Check sheet for the modelled part. Datum: model origin and axes. Units: mm. Round coordinates to 2 decimals unless told otherwise and drop trailing zeros. Order: outer loops, then holes, each group sorted by start corner. A loop starts at its lowest first (then second) coordinate and runs counter-clockwise, first axis right, second up. Notation, with made-up numbers: M 65,38.5 L 85,38.5 A18 cw 85,47.5 Z; hole C -39.75,-37 d5. An arc over 180 degrees is marked long. One line per item, written item: value. Start each with the question number.
(1) Release check for a two-part mould opening along X. For faces 1 (the face through (-3.563, 1.772, -0.791)), 2 (the face through (-2.4, 0, 0.8)), 3 (the face through (0.71, 2.29, 2.24)), 4 (the face through (8.406, 3.575, 3.006)) record: released by +X, released by -X, zero draft, split by the parting line, or undercut.
(2) Thickness scan on L1, parallel to X at y = 3.25, z = 0; L2, parallel to X at y = 2.2, z = 0; L3, parallel to Y at x = 4, z = 2. Record the ranges inside material, lowest first.
(3) Cross-section at D-D, the plane z = 2. Enter the section's corners in (x, y).
(4) Cross-section at C-C, the plane y = 3. Enter the section's corners in (x, z), and give its area (3 significant figures).
(5) Depth check by flat-ended pin: pin 1 Ø3.5 at (x, z) = (8, -1) entering from -Y; pin 2 Ø1 at (y, z) = (1.5, 0.5) entering from -X; pin 3 Ø2 at (x, y) = (4, 1.5) entering from +Z; pin 4 Ø2 at (y, z) = (4, 1.5) entering from +X. Enter the tip coordinate at first touch or a pass-through.
(6) Cross-section at A-A, the plane x = 0. Enter the section's corners in (y, z).
(7) Cross-section at B-B, the plane z = 0. Enter the section's corners in (x, y).
from build123d import *

# Parameters (mm, degrees)
SKETCH1_R           = 3.65
SKETCH1_R_2         = 2.35
BOSS_EXTRUDE1_DEPTH = 4.64
BOSS_EXTRUDE2_START = -2.1
BOSS_EXTRUDE2_DEPTH = 2.1


with BuildPart() as part:
    # Sketch1 → Boss-Extrude1 (new body)
    with BuildSketch(Plane(origin=(0, 0, 0), x_dir=(1, 0, 0), z_dir=(0, 1, 0))):
        with Locations(Location((0, 0, 0), (0, 0, 270))):
            Circle(SKETCH1_R)
        with Locations(Location((0, 0, 0), (0, 0, 270))):
            Circle(SKETCH1_R_2, mode=Mode.SUBTRACT)
    extrude(amount=BOSS_EXTRUDE1_DEPTH)

    # Sketch2 → Boss-Extrude2 (add)
    with BuildSketch(Plane(origin=(0, 4.64, 0), x_dir=(1, 0, 0), z_dir=(0, 1, 0)).offset(BOSS_EXTRUDE2_START)):
        with BuildLine():
            Line((0.283385093, 3.638982397), (16.303738301, 2.391400302))
            ThreePointArc((16.303738301, 2.391400302), (18.500063478, 0), (16.303738301, -2.391400302))
            Line((16.303738301, -2.391400302), (0.283385093, -3.638982397))
            ThreePointArc((0.283385093, -3.638982397), (3.65, 0), (0.283385093, 3.638982397))
        make_face()
    extrude(amount=BOSS_EXTRUDE2_DEPTH)


solid = part.part
Values found:
1. face 1: split by the parting line
1. face 2: zero draft
1. face 3: undercut
1. face 4: released by +X
2. L1: -3.65 to -2.35, 2.35 to 18.5
2. L2: -3.65 to -2.35, 2.35 to 3.65
2. L3: 2.54 to 4.64
3. outline: M -3.05,0 L -1.23,0 L -1.23,4.64 L -3.05,4.64 Z; M 1.23,0 L 3.05,0 L 3.05,2.54 L 17.43,2.54 L 17.43,4.64 L 1.23,4.64 Z
4. outline: M 0.28,-3.64 L 16.3,-2.39 A2.4 ccw 16.3,2.39 L 0.28,3.64 A3.65 ccw long Z; hole C 0,0 d4.7
4. area: 110 mm^2
5. pin 1: y = 2.54
5. pin 2: x = -3.65
5. pin 3: z = 2.08
5. pin 4: x = 18.45
6. outline: M 0,-3.65 L 4.64,-3.65 L 4.64,-2.35 L 0,-2.35 Z; M 0,2.35 L 4.64,2.35 L 4.64,3.65 L 0,3.65 Z
7. outline: M -3.65,0 L -2.35,0 L -2.35,4.64 L -3.65,4.64 Z; M 2.35,0 L 3.65,0 L 3.65,2.54 L 18.5,2.54 L 18.5,4.64 L 2.35,4.64 Z
